Geometry: see drawing. Coordinates: mm, zero at the bounding-box minimum. A direction names the side the tool comes from. Give positions to 0.01 mm unless a question says otherwise; leave off trailing zeros. Write each loop counter-clockwise with the first axis right and the second up, starting at its lowest first coordinate (ties: lowest second). Pieces come first, ordered by that corner, then holes. Notation, with made-up numbers: (-4.75, 40.5) -> (48.25, 40.5) arc R26 cw to (48.25, 56.5) -> close; hole circle Ø7 at (-16.75, 41). An arc over 180 degrees is marked (long way). Answer as a JSON object with one key per item and string values. Group by question number.
Item 1: First-contact query: pin 1 Ø12 at (y, z) = (18, 14) entering from +X; pin 2 Ø1.5 at (y, z) = (3, 60.5) entering from -X; pin 3 Ø3 at (x, y) = (30.5, 13.5) entering from +Z; pin 4 Ø5 at (x, z) = (32, 44.5) entering from +Y. Flat tips, straight axial feed; report the tip coordinate or a pass-through.
Item 2: Section query B-B on z = 54.5. Return the cut outline in (x, y), plus the area to 3 significant figures.
Item 3: Ray query, probe 1 along X at (y, z) = (13.75, 85); probe 2 along Z at (x, y) = (9, 16.5); probe 3 along X at (y, z) = (12, 28) (1 decimal). Return the intervals inside material, ascending. Write a range as from..to.
Item 4: Section query A-A on y = 15.75. Return the cut outline in (x, z), plus the area to 3 significant figures.
Item 5: Access query for the marked faces 1 and 2. Directions: +Z, -Z, +X, -X, +Y, -Y. A direction counts if a zero-diameter tool reaches every point of the face in a straight line with its end or side. Return the directions, or none.
Item 6: Section query C-C on x = 29. Return the cut outline in (y, z), plus the area to 3 significant figures.
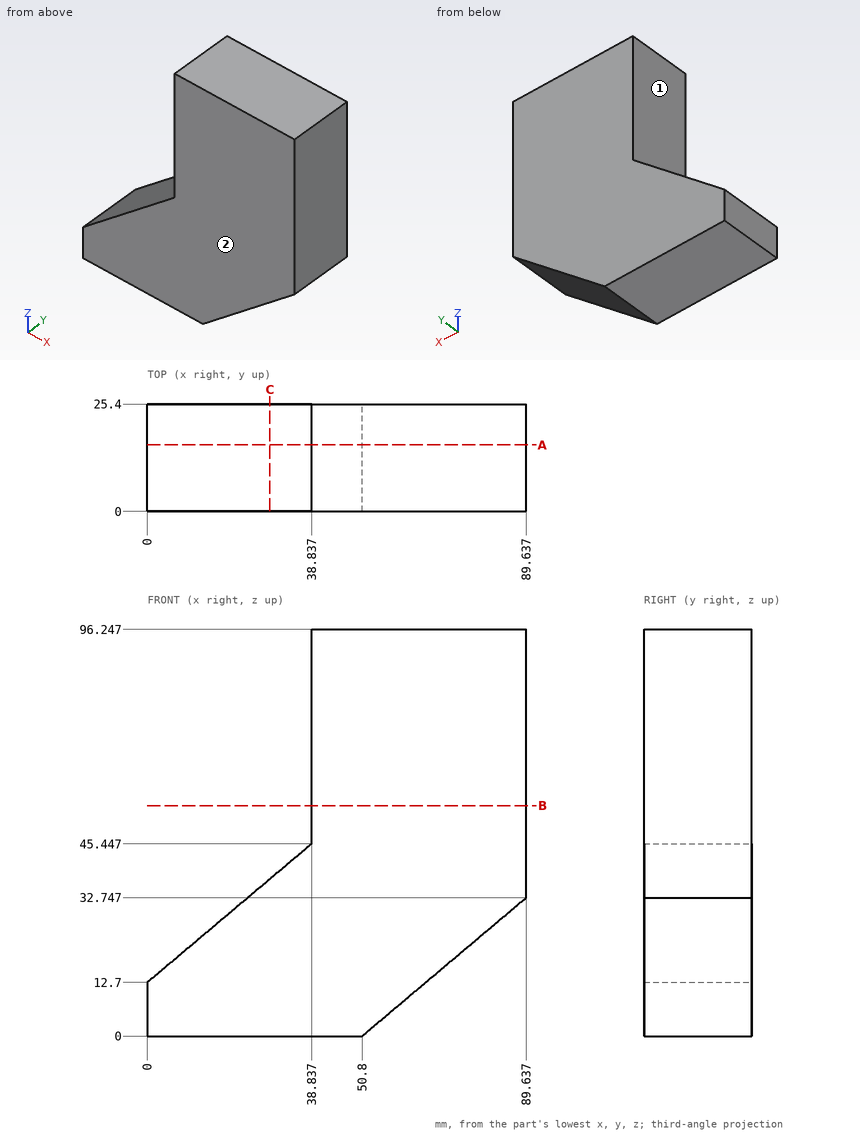
Worked answers:
{
 "1": {"pin 1": "x = 74.52", "pin 2": "x = 38.84", "pin 3": "z = 39.68", "pin 4": "through"},
 "2": {"outline": "(38.84, 0) -> (89.64, 0) -> (89.64, 25.4) -> (38.84, 25.4) -> close", "area": "1,290 mm^2"},
 "3": {"probe 1": "38.84..89.64", "probe 2": "0..20.29", "probe 3": "18.1..84"},
 "4": {"outline": "(0, 0) -> (50.8, 0) -> (89.64, 32.75) -> (89.64, 96.25) -> (38.84, 96.25) -> (38.84, 45.45) -> (0, 12.7) -> close", "area": "5,380 mm^2"},
 "5": {"face 1": "+Z, -X, +Y, -Y", "face 2": "+Z, -Z, +X, -X, -Y"},
 "6": {"outline": "(0, 0) -> (25.4, 0) -> (25.4, 37.15) -> (0, 37.15) -> close", "area": "944 mm^2"}
}
